```python
from build123d import *

# Parameters (mm, degrees)
BOSS_EXTRUDE1_DEPTH  = 15
CUT_EXTRUDE1_DEPTH   = 3.175
MIRROR4_COPY_1_DEPTH = 3.175
FILLET1_R            = 2
FILLET2_R            = 1


with BuildPart() as part:
    # Sketch1 → Boss-Extrude1 (new, symmetric)
    with BuildSketch(Plane.XY):
        with BuildLine():
            Line((-3.1, 3.61543998), (-3.1, 13.7625))
            Line((-3.1, 13.7625), (3.1, 13.7625))
            Line((3.1, 13.7625), (3.1, 3.61543998))
            ThreePointArc((3.1, 3.61543998), (4.326959455, 1.989680408), (4.7625, 0))
            Line((4.7625, 0), (7.7625, 0))
            Line((7.7625, 0), (7.7625, 15.84052737))
            Line((7.7625, 15.84052737), (-7.7625, 15.84052737))
            Line((-7.7625, 15.84052737), (-7.7625, 0))
            Line((-7.7625, 0), (-4.7625, 0))
            ThreePointArc((-4.7625, 0), (-4.326959455, 1.989680408), (-3.1, 3.61543998))
        make_face()
    extrude(amount=BOSS_EXTRUDE1_DEPTH, both=True)

    # Sketch2 → Cut-Extrude1 (cut, symmetric)
    with BuildSketch(Plane.XY.offset(7.5)):
        Polygon((-7.7625, 15.84052737), (-7.7625, 0), (-6.7625, 0), (-6.7625, 14.84052737), (0, 14.84052737), (0, 15.84052737), align=None)
    cut_extrude1 = extrude(amount=CUT_EXTRUDE1_DEPTH, both=True, mode=Mode.SUBTRACT)

    # Mirror3: Cut-Extrude1 across plane
    add(cut_extrude1.mirror(Plane(origin=(0, 0, 0), x_dir=(0, 0, 1), z_dir=(1, 0, 0))), mode=Mode.SUBTRACT)

    # Mirror4: Cut-Extrude1 across plane
    add(cut_extrude1.mirror(Plane.XY), mode=Mode.SUBTRACT)

    # Mirror4 copy 1 sketch → Mirror4 copy 1 (cut, symmetric)
    with BuildSketch(Plane(origin=(0, 0, -7.5), x_dir=(-1, 0, 0), z_dir=(0, 0, -1))):
        Polygon((-7.7625, 15.84052737), (-7.7625, 0), (-6.7625, 0), (-6.7625, 14.84052737), (0, 14.84052737), (0, 15.84052737), align=None)
    extrude(amount=MIRROR4_COPY_1_DEPTH, both=True, mode=Mode.SUBTRACT)

    # Fillet1
    fillet1_edges = [part.edges().sort_by_distance(p)[0] for p in [
        (-6.7625, 14.84052737, 7.5),
        (6.7625, 14.84052737, 7.5),
        (-6.7625, 14.84052737, -7.5),
        (6.7625, 14.84052737, -7.5),
    ]]
    fillet(fillet1_edges, radius=FILLET1_R)

    # Fillet2
    fillet2_edges = [part.edges().sort_by_distance(p)[0] for p in [
        (-6.7625, 0, 7.5),
        (6.7625, 0, 7.5),
        (-6.7625, 0, -7.5),
        (6.7625, 0, -7.5),
    ]]
    fillet(fillet2_edges, radius=FILLET2_R)


solid = part.part
```
Geometry check sheet. Reference: the model listing, model coordinates, mm. A direction names the side the tool comes from. Give positions to 0.01 mm unless a question says otherwise; leave off trailing zeros. Order: outer loops, then holes, each group sorted by start corner. A loop starts at its lowest first (then second) coordinate and runs counter-clockwise, first axis right, second up. Notation, with made-up numbers: (58, 37) - (77, 37) arc R9 cw to (77, 51) - close; hole circle Ø3 at (-13, 44.25). An arc over 180 degrees is marked (long way). Answer in a Markdown table with one row per item. Add a question column.
Q1. Material ranges on probe 1 along Z at (x, y) = (6.75, 13.5) (3 decimals); probe 2 along X at (y, z) = (4.5, 11.25); probe 3 along X at (y, z) = (4, 7.5), recorded low to high. Write a range as from..to.
Q2. Cross-section at D-D, the plane z = 3.25. Enter the section's corners in (x, y) (1 decimal), then the cut area to 3 significant figures.
Q3. Cross-section at C-C, the plane x = -0.25. Enter the section's corners in (y, z) (1 decimal), then the cut area to 3 significant figures.
Q4. Mould release check, pull along Z, two halves, no side actions. Record for faces 4 (the cylindrical face through (6.19, 14.24, 7.54)), 5 (the flat face through (3.3, 8, -15)), 6 (the flat face through (0, 15.841, 0)): pulls with the +Z half, pulls with the -Z half, needs draft (parallel to the pull), parting line crosses it, or undercut.
Q5. Cross-section at A-A, the plane y = 8.75. Enter the section's corners in (x, z) (1 decimal), then the cut area to 3 significant figures.
Q6. Tool access check on faces 1 (the flat face through (6.762, 7, -8)), 2 (the cylindrical face through (6.477, 0.301, -7.544)), 3 (the cylindrical face through (-6.16, 14.27, -7.54)). Record the directions out of +Z, -Z, +X, -X, +Y, -Y that give a thin tool (end or side, any length) a straight path to the whole face; none if there is none.
Q7. Cross-section at B-B, the plane z = 6.25. Enter the section's corners in (x, y) (1 decimal).
Q8. Gauge pin test, flat ends, axial feed: pin 1 (1.5 mm diameter, centred on y = 4.5, z = 7.5, fed in from -X); pin 2 (3 mm diameter, centred on x = 1.5, z = 8, fed in from +Y); pin 3 (4 mm diameter, centred on x = -0.5, z = 9, fed in from -Y). Record the tip position at first contact, or that the pin passes through.
Check values:
| question | item | result |
|---|---|---|
| 1 | probe 1 | z = -15..-10.675, -4.325..4.325, 10.675..15 |
| 1 | probe 2 | x = -7.76..-3.1, 3.1..7.76 |
| 1 | probe 3 | x = -6.76..-3.1, 3.1..6.76 |
| 2 | outline | (-7.8, 0) - (-4.8, 0) arc R4.8 cw to (-3.1, 3.6) - (-3.1, 13.8) - (3.1, 13.8) - (3.1, 3.6) arc R4.8 cw to (4.8, 0) - (7.8, 0) - (7.8, 15.8) - (-7.8, 15.8) - close |
| 2 | area | 152 mm^2 |
| 3 | outline | (13.8, -15) - (15.8, -15) - (15.8, -10.7) - (14.8, -10.7) - (14.8, -4.3) - (15.8, -4.3) - (15.8, 4.3) - (14.8, 4.3) - (14.8, 10.7) - (15.8, 10.7) - (15.8, 15) - (13.8, 15) - close |
| 3 | area | 49.6 mm^2 |
| 4 | face 4 | undercut |
| 4 | face 5 | pulls with the -Z half |
| 4 | face 6 | needs draft |
| 5 | outline | (-7.8, -15) - (-3.1, -15) - (-3.1, 15) - (-7.8, 15) - (-7.8, 10.7) - (-6.8, 10.7) - (-6.8, 4.3) - (-7.8, 4.3) - (-7.8, -4.3) - (-6.8, -4.3) - (-6.8, -10.7) - (-7.8, -10.7) - close; (3.1, -15) - (7.8, -15) - (7.8, -10.7) - (6.8, -10.7) - (6.8, -4.3) - (7.8, -4.3) - (7.8, 4.3) - (6.8, 4.3) - (6.8, 10.7) - (7.8, 10.7) - (7.8, 15) - (3.1, 15) - close |
| 5 | area | 254 mm^2 |
| 6 | face 1 | +X, +Y, -Y |
| 6 | face 2 | +X, -Y |
| 6 | face 3 | -X, +Y |
| 7 | outline | (-6.8, 1) arc R1 ccw to (-5.8, 0) - (-4.8, 0) arc R4.8 cw to (-3.1, 3.6) - (-3.1, 13.8) - (3.1, 13.8) - (3.1, 3.6) arc R4.8 cw to (4.8, 0) - (5.8, 0) arc R1 ccw to (6.8, 1) - (6.8, 12.8) arc R2 ccw to (4.8, 14.8) - (-4.8, 14.8) arc R2 ccw to (-6.8, 12.8) - close |
| 8 | pin 1 | stops at x = -6.76 |
| 8 | pin 2 | stops at y = 14.84 |
| 8 | pin 3 | stops at y = 13.76 |
